Input: part model. Units: mm. Frame: model coordinates. Face numbers are marked on the shaded views. A direction names the side the tool comes from. Give positions to 0.01 mm unless a question says otherwise; leave off trailing zeros. Loops run counter-clockwise (first coordinate to the right, second up) from the corner with the lowest first, then second, coordinate; pieces in that order, holes last. Notation, with made-up numbers: M -27,62 L -17,62 A26 ccw -17,95 Z; hole C 17.25,53 d6. An arc over 180 degrees is marked long. Answer as a JSON object with one key per item and string values. Group by question number.
1) Access query for the marked faces 1 and 2. Directions: +Z, -Z, +X, -X, +Y, -Y. A direction counts if a zero-diameter tool reaches every point of the face in a straight line with its end or side. Return the directions, or none.
2) Section query B-B on z = 28. Return loops of the section in (x, y) (3 decimals), plus the area to 3 significant figures.
3) Section query C-C on y = -14.5. Return loops of the section in (x, z).
4) First-contact query: P1, Ø5, axis at x = -3.5, y = 15, coming from the -Z side; P2, Ø5, axis at y = 2.5, z = 10.5, coming from the +X side; P3, Ø0.9, axis at x = 43.5, z = 10.5, coming from the +Y side. Flat tips, straight axial feed; report the tip coordinate or a pass-through.
5) Ray query, L1, parallel to Y at x = -39, z = 10 (3 decimals); L2, parallel to X at y = -24, z = 23; L3, parallel to X at y = 4.5, z = 17. Return the intervals inside material, ascending.
6) Section query A-A on x = 19. Return loops of the section in (y, z) (3 decimals).
from build123d import *

# Parameters (mm, degrees)
SKETCH1_R           = 1.375
SKETCH1_W           = 53.678190842
SKETCH1_H           = 4.106512076
SKETCH1_W_2         = 1.875741611
SKETCH1_H_2         = 11.459220881
SKETCH1_W_3         = 17.06705209
BOSS_EXTRUDE1_DEPTH = 35


with BuildPart() as part:
    # Sketch1 → Boss-Extrude1 (new body)
    with BuildSketch(Plane.XY):
        with BuildLine():
            Line((39.5, 28), (-39.5, 28))
            ThreePointArc((-39.5, 28), (-41.621320344, 27.121320344), (-42.5, 25))
            Line((-42.5, 25), (-42.5, -25))
            ThreePointArc((-42.5, -25), (-41.621320344, -27.121320344), (-39.5, -28))
            Line((-39.5, -28), (39.5, -28))
            ThreePointArc((39.5, -28), (41.621320344, -27.121320344), (42.5, -25))
            Line((42.5, -25), (42.5, 9.398790598))
            Line((42.5, 9.398790598), (25.43294791, 9.398790598))
            Line((25.43294791, 9.398790598), (25.43294791, 20.858011479))
            Line((25.43294791, 20.858011479), (42.5, 20.858011479))
            Line((42.5, 20.858011479), (42.5, 25))
            ThreePointArc((42.5, 25), (41.621320344, 27.121320344), (39.5, 28))
        make_face()
        with Locations((-39, -24.5)):
            Circle(SKETCH1_R, mode=Mode.SUBTRACT)
        with Locations((19, -24.5)):
            Circle(SKETCH1_R, mode=Mode.SUBTRACT)
        with Locations((-39, 24.5)):
            Circle(SKETCH1_R, mode=Mode.SUBTRACT)
        with Locations((-10.129653796, 24.707102416)):
            Rectangle(SKETCH1_W, SKETCH1_H, mode=Mode.SUBTRACT)
        with Locations((19, 24.5)):
            Circle(SKETCH1_R, mode=Mode.SUBTRACT)
        with Locations((-10.129653796, 24.707102416)):
            Rectangle(SKETCH1_W, SKETCH1_H)
        with Locations((43.437870805, 15.128401039)):
            Rectangle(SKETCH1_W_2, SKETCH1_H_2)
        with Locations((33.966473955, 15.128401039)):
            Rectangle(SKETCH1_W_3, SKETCH1_H_2)
    extrude(amount=BOSS_EXTRUDE1_DEPTH)


solid = part.part
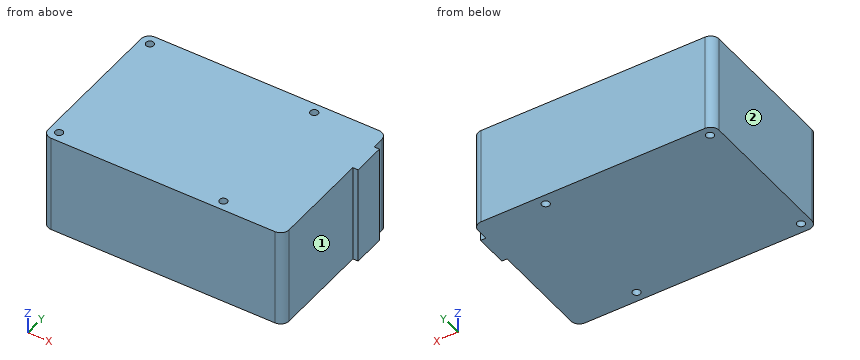
Output:
{
 "1": {"face 1": "+Z, -Z, +X, -Y", "face 2": "+Z, -Z, -X, +Y, -Y"},
 "2": {"outline": "M -42.5,-25 A3 ccw -39.5,-28 L 39.5,-28 A3 ccw 42.5,-25 L 42.5,9.399 L 44.376,9.399 L 44.376,20.858 L 42.5,20.858 L 42.5,25 A3 ccw 39.5,28 L -39.5,28 A3 ccw -42.5,25 Z; hole C -39,-24.5 d2.75; hole C -39,24.5 d2.75; hole C 19,-24.5 d2.75; hole C 19,24.5 d2.75", "area": "4,750 mm^2"},
 "3": {"outline": "M -42.5,0 L 42.5,0 L 42.5,35 L -42.5,35 Z"},
 "4": {"P1": "stops at z = 0", "P2": "stops at x = 42.5", "P3": "stops at y = 20.86"},
 "5": {"L1": "y = -28 to -25.875, -23.125 to 23.125, 25.875 to 28", "L2": "x = -42.5 to -40.28, -37.72 to 17.72, 20.28 to 42.5", "L3": "x = -42.5 to 42.5"},
 "6": {"outline": "M -28,0 L -25.875,0 L -25.875,35 L -28,35 Z; M -23.125,0 L 23.125,0 L 23.125,35 L -23.125,35 Z; M 25.875,0 L 28,0 L 28,35 L 25.875,35 Z"}
}
